Can you work these out from the model? Positions are in its coordinate system, mm. A direction names the side the tool comes from. Give positions to 0.01 mm unless a question says otherwise; leave off trailing zeros. Write each loop counter-clockwise with the first axis right and the second up, starting at its lowest first coordinate (ties: lowest second). Pieces come first, ordered by that corner, then holes.
1. On a 3-axis mill with a long thin cutter (end or side, diameter ignored), from which of +Z, -Z, +X, -X, +Y, -Y can I reach the whole of each face in a straight line? I mean faces 4 (the flat face through (-2, 18, 50.8)), 5 (the flat face through (0, 18, 25)). Say none if no direction works.
2. Suppose I cut it at C-C (x = 27). Please give me the cut outline in (y, z) (3 decimals), and give its area (3 significant figures).
3. Suppose I cut it at D-D (y = 14). Please give me the cut outline in (x, z) (3 decimals), and give its area (3 significant figures).
4. Suppose I cut it at A-A (y = 22.86). Please give me the cut outline in (x, z) (3 decimals), and give its area (3 significant figures).
5. If I drill on probe 1 along X at (y, z) = (15.5, 35.5) (3 decimals); probe 2 along Z at (x, y) = (-1, 11.5), over which ranges is the centre line in solid material (lowest first)?
6. Thinking about a two-plate mould opening in Z: for faces 1 (the cylindrical face through (17.98, -1.57, 36.01)), 2 (the flat face through (47.625, -2, 13)), 3 (the flat face through (-2, 18, 0)), which applies, pulls with the +Z half, pulls with the -Z half, needs draft (parallel to the pull), parting line crosses it, or undercut?
7. Suppose I cut it at B-B (z = 30.5). Please give me the cut outline in (x, y) (3 decimals), and give its area (3 significant figures).
8. I'm going to push flat-ended pins straight in: pin 1 (6 mm diameter, centred on y = 22.86, z = 9.525, fed in from +X); pin 2 (10.5 mm diameter, centred on y = 25, z = 26, fed in from +X); pin 3 (6 mm diameter, centred on x = 34, z = 39.5, fed in from +Y); pin 4 (9 mm diameter, centred on x = 35.15, z = 4.19, fed in from -Y) (3 decimals). Where does each tip first touch, or does it pass through?
Autodesk Inventor part; units mm, degrees
ref_plane "YZ Plane" through (0, 0, 0) normal (1, 0, 0) x (0, 1, 0)
ref_plane "XZ Plane" through (0, 0, 0) normal (0, 1, 0) x (-1, 0, 0)
ref_plane "XY Plane" through (0, 0, 0) normal (0, 0, 1) x (1, 0, 0)
sketch "Sketch1" plane through (0, 0, 0) normal (0, 0, 1) x (1, 0, 0)
  line L0 (0, 0) -> (47.625, 0)
  line L1 (47.625, 0) -> (47.625, -3.175)
  line L2 (47.625, -3.175) -> (-3.175, -3.175)
  line L3 (-3.175, -3.175) -> (-3.175, 47.625)
  line L4 (-3.175, 47.625) -> (0, 47.625)
  line L5 (0, 47.625) -> (0, 0)
  dimension "d14" = 50.8
  dimension "d15" = 3.175
extrude "Extrusion1" add sketch "Sketch1" along normal blind 50.8
sketch "Sketch2" plane through (0, 0, 0) normal (1, 0, 0) x (0, 0, -1)
  circle A0 centre (-9.525, 22.86) radius 3.3734
  circle A1 centre (-36.5125, 22.86) radius 3.3734
  line L0 (0, 0) -> (-50.8, 0)
  line L1 (0, 47.625) -> (0, 0)
  line L2 (-50.8, 0) -> (-50.8, 47.625)
  dimension "d6" = 6.7469
  dimension "d7" = 6.7469
  dimension "d8" = 22.86
  dimension "d9" = 22.86
  dimension "d16" = 14.2875
  dimension "d17" = 41.275
extrude "Extrusion2" cut sketch "Sketch2" against normal blind 3.175
sketch "Sketch3" plane through (0, 0, 0) normal (0, 1, 0) x (1, 0, 0)
  line L0 (0, -50.8) -> (-3.175, -50.8)
  line L1 (-3.175, -50.8) -> (47.625, -39.0719)
  line L2 (47.625, -50.8) -> (0, -50.8)
  circle A0 centre (35.1496, -4.1861) radius 3.3734
  circle A1 centre (18.7171, -32.7117) radius 3.3782
  line L3 (-3.175, 0) -> (-3.175, -50.8)
  line L4 (-3.175, -50.8) -> (-14.6025, -1.302) construction
  line L5 (47.625, 0) -> (47.625, -50.8)
  line L6 (47.625, 0) -> (47.625, -50.8)
  line L7 (47.625, -39.0719) -> (47.625, -50.8)
  line L8 (47.625, -50.8) -> (-3.175, -50.8)
  line L9 (-3.175, 0) -> (0, 0)
  line L10 (-3.175, 0) -> (47.625, 11.7281)
  line L11 (47.625, 11.7281) -> (47.625, 0)
  line L12 (47.625, 0) -> (-3.175, 0)
  line L13 (0, 0) -> (0, -50.8)
  dimension "d18" = 13
  dimension "d19" = 6.7469
  dimension "d20" = 6.7564
  dimension "d21" = 12.7
  dimension "d22" = 50.8
  dimension "d23" = 25.4
  dimension "d24" = 21.8921
  dimension "d26" = 12.7
  dimension "d35" = 47.8282
  dimension "d36" = 12.4754
  dimension "d37" = 18.7171
extrude "Extrusion3" cut sketch "Sketch3" against normal blind 3.175 contours L13 L1 L5 L2 | L0 L1 L13 | A0 | A1
extrude "Extrusion4" add sketch "Sketch3" against normal blind 3.175 contours L10 L11 L12 L9
sketch "Sketch4" plane through (0, 0, 0) normal (1, 0, 0) x (0, 0, -1)
  line L0 (-50.8, 0) -> (-50.8, 47.625)
  line L1 (0, 47.625) -> (0, 0)
  line L2 (-50.8, 47.625) -> (0, 47.625)
  line L3 (0, 47.625) -> (0, 35.56)
  line L4 (0, 35.56) -> (-50.8, 35.56)
  line L5 (-50.8, 35.56) -> (-50.8, 47.625)
  dimension "d32" = 12.065
extrude "Extrusion5" cut sketch "Sketch4" against normal blind 3.175
properties part number "rail gusset" material "Aluminum 6061"
Checks:
1. face 4: +Z, +X, -X, +Y, -Y
1. face 5: +Z, -Z, +X, +Y
2. outline: (-3.175, -6.966) - (0, -6.966) - (0, 43.834) - (-3.175, 43.834) - close
2. area: 161 mm2
3. outline: (-3.175, 0) - (0, 0) - (0, 50.8) - (-3.175, 50.8) - close
3. area: 161 mm2
4. outline: (-3.175, 0) - (0, 0) - (0, 6.152) - (-3.175, 6.152) - close; (-3.175, 12.898) - (0, 12.898) - (0, 33.139) - (-3.175, 33.139) - close; (-3.175, 39.886) - (0, 39.886) - (0, 50.8) - (-3.175, 50.8) - close
4. area: 118 mm2
5. probe 1: x = -3.175 to 0
5. probe 2: z = 0 to 50.8
6. face 1: undercut
6. face 2: needs draft
6. face 3: pulls with the -Z half
7. outline: (-3.175, -3.175) - (16.164, -3.175) - (16.164, 0) - (0, 0) - (0, 35.56) - (-3.175, 35.56) - close; (21.271, -3.175) - (47.625, -3.175) - (47.625, 0) - (21.271, 0) - close
7. area: 258 mm2
8. pin 1: passes through
8. pin 2: stops at x = 0
8. pin 3: stops at y = 0
8. pin 4: stops at y = -3.175
